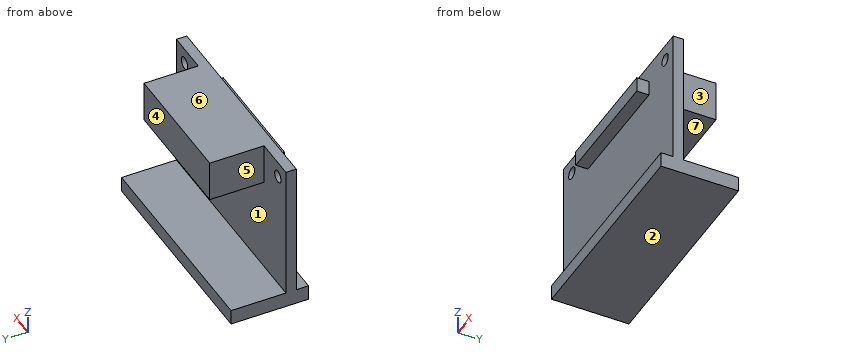
```python
from build123d import *

# Parameters (mm, degrees)
SKETCH1_W           = 35
SKETCH1_H           = 25
BOSS_EXTRUDE1_DEPTH = 1.7
SKETCH2_W           = 21
SKETCH2_H           = 6.8
BOSS_EXTRUDE2_DEPTH = 8.9
SKETCH3_W           = 35
SKETCH3_H           = 2.5
BOSS_EXTRUDE3_DEPTH = 9
SKETCH4_W           = 35
SKETCH4_H           = 2.5
SKETCH4_W_2         = 19.5
BOSS_EXTRUDE4_DEPTH = 2
CUT_EXTRUDE1_REACH  = 25.313
SKETCH5_R           = 1


with BuildPart() as part:
    # Sketch1 → Boss-Extrude1 (new body)
    with BuildSketch(Plane(origin=(0, 0, 0), x_dir=(1, 0, 0), z_dir=(0, 1, 0))):
        Rectangle(SKETCH1_W, SKETCH1_H)
    extrude(amount=BOSS_EXTRUDE1_DEPTH)

    # Sketch2 → Boss-Extrude2 (add)
    with BuildSketch(Plane(origin=(0, 1.7, 0), x_dir=(1, 0, 0), z_dir=(0, 1, 0))):
        with Locations((0, -9.1)):
            Rectangle(SKETCH2_W, SKETCH2_H)
    extrude(amount=BOSS_EXTRUDE2_DEPTH)

    # Sketch3 → Boss-Extrude3 (add)
    with BuildSketch(Plane(origin=(0, 1.7, 0), x_dir=(1, 0, 0), z_dir=(0, 1, 0))):
        with Locations((0, 11.25)):
            Rectangle(SKETCH3_W, SKETCH3_H)
    extrude(amount=BOSS_EXTRUDE3_DEPTH)

    # Sketch4 → Boss-Extrude4 (add)
    with BuildSketch(Plane.XZ):
        with Locations((0, -11.25)):
            Rectangle(SKETCH4_W, SKETCH4_H)
        with Locations((0, 8.25)):
            Rectangle(SKETCH4_W_2, SKETCH4_H)
    extrude(amount=BOSS_EXTRUDE4_DEPTH)

    # Sketch5 → Cut-Extrude1 (cut, up to next)
    with BuildSketch(Plane(origin=(0, 1.7, 0), x_dir=(1, 0, 0), z_dir=(0, 1, 0)), mode=Mode.PRIVATE) as cut_extrude1_sk1:
        with Locations(Location((14.9, -9.9, 0), (0, 0, 270))):
            Circle(SKETCH5_R)
    cut_extrude1_tool1 = extrude(cut_extrude1_sk1.sketch, amount=-CUT_EXTRUDE1_REACH, mode=Mode.PRIVATE) & part.part
    # Sketch5 → Cut-Extrude1 (cut, up to next)
    with BuildSketch(Plane(origin=(0, 1.7, 0), x_dir=(1, 0, 0), z_dir=(0, 1, 0)), mode=Mode.PRIVATE) as cut_extrude1_sk2:
        with Locations(Location((-14.9, -9.9, 0), (0, 0, 270))):
            Circle(SKETCH5_R)
    cut_extrude1_tool2 = extrude(cut_extrude1_sk2.sketch, amount=-CUT_EXTRUDE1_REACH, mode=Mode.PRIVATE) & part.part
    add(cut_extrude1_tool1.solids().sort_by_distance((14.9, 1.7, 9.9))[0], mode=Mode.SUBTRACT)
    add(cut_extrude1_tool2.solids().sort_by_distance((-14.9, 1.7, 9.9))[0], mode=Mode.SUBTRACT)


solid = part.part
```
The listing builds one solid part. Answer for the finished solid, in the listing's coordinates (mm). Face numbers are marked on the shaded views. A direction names the side the tool comes from. Give positions to 0.01 mm unless a question says otherwise; leave off trailing zeros. Order: outer loops, then holes, each group sorted by start corner. A loop starts at its lowest first (then second) coordinate and runs counter-clockwise, first axis right, second up.
Item 1: Given pin 1 Ø4 at (x, z) = (10.5, 10) entering from +Y; pin 2 Ø4 at (y, z) = (4, 2.5) entering from +X; pin 3 Ø5.5 at (y, z) = (7, 9) entering from -X; pin 4 Ø5.5 at (y, z) = (7, 9) entering from +X, each flat-ended and moving along its own axis, determine where each tip first touches the part or whether it passes through.
From the geometry:
pin 1: stops at y = 10.6
pin 2: passes through
pin 3: stops at x = -10.5
pin 4: stops at x = 10.5
Item 2: Find the intervals of material crossed by probe 1 along X at (y, z) = (0.85, 9.9); probe 2 along Z at (x, y) = (-9, 1.75); probe 3 along X at (y, z) = (1.75, 10.75), in increasing order.
From the geometry:
probe 1: x = -17.5 to -15.9, -13.9 to 13.9, 15.9 to 17.5
probe 2: z = -12.5 to -10, 5.7 to 12.5
probe 3: x = -10.5 to 10.5
Item 3: The part is cut by section B-B, the plane z = 9.9. Give the vertices of the cut face in (x, y), and give its area (3 significant figures).
From the geometry:
outline: (-17.5, 0) - (-15.9, 0) - (-15.9, 1.7) - (-17.5, 1.7) - close; (-13.9, 0) - (13.9, 0) - (13.9, 1.7) - (10.5, 1.7) - (10.5, 10.6) - (-10.5, 10.6) - (-10.5, 1.7) - (-13.9, 1.7) - close; (15.9, 0) - (17.5, 0) - (17.5, 1.7) - (15.9, 1.7) - close
area: 240 mm2
Item 4: Which of the six approach directions +Z, -Z, +X, -X, +Y, -Y give full straight-line access (tool end or side, diameter ignored) to the marked faces 4, 5, 6 and 7?
From the geometry:
face 4: +Z, +X, -X, +Y
face 5: +Z, -X, +Y
face 6: +Z, +X, -X, +Y, -Y
face 7: +X, -X, +Y
Item 5: The part is cut by section D-D, the plane x = 1. Give the vertices of the cut face in (y, z), and give its area (3 significant figures).
From the geometry:
outline: (-2, -12.5) - (10.7, -12.5) - (10.7, -10) - (1.7, -10) - (1.7, 5.7) - (10.6, 5.7) - (10.6, 12.5) - (0, 12.5) - (0, 9.5) - (-2, 9.5) - (-2, 7) - (0, 7) - (0, -10) - (-2, -10) - close
area: 136 mm2
Item 6: The part is cut by section A-A, the plane x = -14.9. Give the vertices of the cut face in (y, z), and give its area (3 significant figures).
From the geometry:
outline: (-2, -12.5) - (10.7, -12.5) - (10.7, -10) - (1.7, -10) - (1.7, 8.9) - (0, 8.9) - (0, -10) - (-2, -10) - close; (0, 10.9) - (1.7, 10.9) - (1.7, 12.5) - (0, 12.5) - close
area: 66.6 mm2
Item 7: The part is cut by section C-C, the plane y = 8. Give the vertices of the cut face in (x, z).
From the geometry:
outline: (-17.5, -12.5) - (17.5, -12.5) - (17.5, -10) - (-17.5, -10) - close; (-10.5, 5.7) - (10.5, 5.7) - (10.5, 12.5) - (-10.5, 12.5) - close
Item 8: For a pull along Z with two mould halves and no side action, classify the marked faces 1, 2 and 3 as pulls with the +Z half, pulls with the -Z half, needs draft (parallel to the pull), parting line crosses it, or undercut.
From the geometry:
face 1: undercut
face 2: pulls with the -Z half
face 3: needs draft
